from build123d import *

# Parameters (mm, degrees)
F3_DEPTH = 88.9
F4_R     = 6


with BuildPart() as f1:
    # F0 (on Top) → F1 (revolve)
    with BuildSketch(Plane.XY):
        with BuildLine():
            Line((0, 100), (0, 0))
            Line((0, 0), (10, 0))
            ThreePointArc((10, 0), (21.038486, 49.472306), (17, 100))
            Line((17, 100), (0, 100))
        make_face()
    revolve(axis=Axis((0, 50, 0), (0, 1, 0)))

    # F2 (on face) → F3 (cut)
    with BuildSketch(Plane.XZ):
        with BuildLine():
            Line((0, 3.1), (-0.226697, 3.492651))
            ThreePointArc((-0.226697, 3.492651), (-2.057248, 2.831559), (-3.251655, 1.29489))
            Line((-3.251655, 1.29489), (-2.948275, 0.957953))
            Line((-2.948275, 0.957953), (-3.391761, 0.863687))
            ThreePointArc((-3.391761, 0.863687), (-3.328698, -1.081559), (-2.23633, -2.692365))
            Line((-2.23633, -2.692365), (-1.822134, -2.507953))
            Line((-1.822134, -2.507953), (-1.869527, -2.958863))
            ThreePointArc((-1.869527, -2.958863), (0, -3.5), (1.869527, -2.958863))
            Line((1.869527, -2.958863), (1.822134, -2.507953))
            Line((1.822134, -2.507953), (2.23633, -2.692365))
            ThreePointArc((2.23633, -2.692365), (3.328698, -1.081559), (3.391761, 0.863687))
            Line((3.391761, 0.863687), (2.948275, 0.957953))
            Line((2.948275, 0.957953), (3.251655, 1.29489))
            ThreePointArc((3.251655, 1.29489), (2.057248, 2.831559), (0.226697, 3.492651))
            Line((0.226697, 3.492651), (0, 3.1))
        make_face()
    extrude(amount=-F3_DEPTH, mode=Mode.SUBTRACT)

    # F4
    f4_edges = [f1.edges().sort_by_distance(p)[0] for p in [
        (-10, 0, 0),
        (-17, 100, 0),
    ]]
    fillet(f4_edges, radius=F4_R)


solid = f1.part
Here's how the part is built. I have some questions about the finished solid (model axes, mm). A direction names the side the tool comes from. Coordinates: 2 decimals unless noted, no trailing zeros.
Item 1: If we mould it in two halves opening along X, with no side actions, what happens to faces 1 (the face through (0, 43.8, -3.5)), 2 (the face through (0, 100, 0)), 3 (the face through (3.32, 43.83, -1.11))? For each: +X half, -X half, draft (parallel to the pull), parting line (faces both ways), or undercut.
Result sheet:
face 1: undercut
face 2: draft
face 3: undercut
Item 2: I need wall thicknesses on line 1 (X direction, y = 60.5, z = 5.5); line 2 (X direction, y = 28, z = 15); line 3 (X direction, y = 56, z = -2). Which ranges of each line are inside material? Lowest first, please.
Result sheet:
line 1: x = -20.73 to 20.73
line 2: x = -10.22 to 10.22
line 3: x = -21.28 to -2.87, 2.87 to 21.28
Item 3: For P1, Ø3, axis at y = 12.5, z = -4, coming from the +X side; P2, Ø5, axis at y = 58.5, z = -6, coming from the +X side; P3, Ø2, axis at x = -12.5, y = 77.5, coming from the -Z side, each with a flat end and sliding along its axis, tell me the tip position at first contact or that it passes through.
Result sheet:
P1: stops at x = 14.31
P2: stops at x = 21.14
P3: stops at z = -17.2
Item 4: For faces 4 (the face through (-2.03, 43.83, 2.85)), 5 (the face through (-3, 0, 3)), which set-ups out of +Z, -Z, +X, -X, +Y, -Y let a thin tool reach every point of the face, with its end or its side?
Result sheet:
face 4: -Y
face 5: +Z, -Z, +X, -X, -Y
